Autodesk Inventor part; units mm, degrees
ref_plane "YZ Plane" through (0, 0, 0) normal (1, 0, 0) x (0, 1, 0)
ref_plane "XZ Plane" through (0, 0, 0) normal (0, 1, 0) x (-1, 0, 0)
ref_plane "XY Plane" through (0, 0, 0) normal (0, 0, 1) x (1, 0, 0)
sketch "Szkic2" plane through (0, 0, 0) normal (0, 1, 0) x (-1, 0, 0)
  line L0 (0, 0) -> (-15, 0) construction
  line L1 (-15, 0) -> (-15, 20)
  line L2 (-15, 20) -> (0, 20)
  line L3 (-15, 0) -> (-15, -20)
  line L4 (-15, -20) -> (0, -20)
  line L5 (0, -20) -> (0, 20) construction
  line L6 (15, 0) -> (15, 20)
  line L7 (15, 20) -> (0, 20)
  line L8 (15, -20) -> (0, -20)
  line L9 (15, 0) -> (15, -20)
  line L10 (15, 0) -> (13, 0) construction
  line L11 (0, 20) -> (0, 18) construction
  line L12 (0, 18) -> (13, 18)
  line L13 (13, 18) -> (13, 0)
  line L14 (0, 18) -> (-13, 18)
  line L15 (-13, 18) -> (-13, 0)
  line L16 (0, -18) -> (13, -18)
  line L17 (13, -18) -> (13, 0)
  line L18 (-13, -18) -> (-13, 0)
  line L19 (0, -18) -> (-13, -18)
  point P0 (-7.5, -20)
  point P1 (15, -10)
  dimension "d18" = 40
  dimension "d19" = 30
  dimension "d22" = 2
  dimension "d23" = 2
extrude "Wyciągnięcie proste4" add sketch "Szkic2" along normal blind 1200
sketch "Szkic3" plane through (15, 0, -20) normal (0, 0, -1) x (-1, 0, 0)
  line L0 (0, 1200) -> (0, 1180) construction
  line L1 (0, 0) -> (0, 1200)
  line L2 (0, 1180) -> (12, 1180) construction
  line L3 (12, 1180) -> (12, 0)
  line L4 (0, 0) -> (0, 1200)
  line L5 (0, 0) -> (0, 20)
  line L6 (0, 20) -> (12, 20)
  point P0 (15, 0)
  dimension "d26" = 20
  dimension "d27" = 12
  dimension "d76" = 1180
  dimension "d77" = 20
hole "Otwór1" at (3, 1180, -20) at (3, 20, -20) direction (0, 0, 1) diameter 8 depth 10 tip angle 118
sketch "Szkic4" plane through (15, 0, 20) normal (1, 0, 0) x (0, 0, -1)
  line L0 (40, 0) -> (0, 0)
  line L1 (0, 0) -> (10, 0)
  line L2 (40, 0) -> (30, 0)
  line L3 (0, 0) -> (0, 31)
  line L4 (0, 0) -> (0, 1200)
  line L5 (0, 31) -> (10, 31)
  line L6 (40, 0) -> (40, 1200)
  line L7 (40, 0) -> (40, 31)
  line L8 (30, 31) -> (40, 31)
  line L9 (40, 31) -> (40, 0)
  line L10 (0, 0) -> (0, 40)
  line L11 (20, 0) -> (20, 13)
  dimension "d35" = 10
  dimension "d36" = 10
  dimension "d37" = 31
  dimension "d38" = 20
  dimension "d39" = 31
  dimension "d40" = 10
  dimension "d41" = 40
  dimension "d42" = 13
hole "Otwór2" at (15, 31, 10) at (15, 31, -10) at (15, 13, 0) direction (-1, 0, 0) diameter 8 depth 8.25 tip angle 118
sketch "Szkic5" plane through (15, 0, 20) normal (1, 0, 0) x (0, 0, -1)
  line L0 (40, 0) -> (0, 0)
  line L1 (0, 0) -> (0, 45)
  line L2 (0, 0) -> (0, 1200)
  line L3 (0, 45) -> (20, 45)
  point P0 (20, 0)
  dimension "d50" = 45
hole "Otwór3" at (15, 45, 0) direction (-1, 0, 0) diameter 5 depth 8 tip angle 118
sketch "Szkic6" plane through (15, 0, 20) normal (1, 0, 0) x (0, 0, -1)
  line L0 (0, 0) -> (0, 1200)
  circle A0 centre (20, 45) radius 2.5
  line L1 (0, 45) -> (3, 45)
  line L2 (3, 45) -> (3, 245)
  line L3 (3, 245) -> (3, 445)
  line L4 (3, 445) -> (3, 645)
  line L5 (3, 645) -> (3, 845)
  line L6 (3, 845) -> (3, 1035)
  line L7 (40, 1200) -> (0, 1200)
  line L8 (20, 0) -> (20, 1200)
  line L9 (0, 1165) -> (4, 1165)
  point P0 (2, 1200)
  point P1 (37, 45)
  point P2 (37, 245)
  point P3 (37, 445)
  point P4 (37, 645)
  point P5 (37, 845)
  point P6 (37, 1035)
  point P7 (36, 1165)
  dimension "d58" = 20
  dimension "d59" = 3
  dimension "d60" = 200
  dimension "d61" = 200
  dimension "d62" = 200
  dimension "d63" = 200
  dimension "d64" = 190
  dimension "d73" = 35
  dimension "d75" = 4
hole "Otwór4" at (15, 45, 17) at (15, 245, 17) at (15, 445, 17) at (15, 645, 17) at (15, 845, 17) at (15, 1035, 17) at (15, 1165, 16) at (15, 1165, -16) at (15, 1035, -17) at (15, 845, -17) at (15, 645, -17) at (15, 445, -17) at (15, 245, -17) at (15, 45, -17) direction (-1, 0, 0) diameter 2.5 depth 8 tip angle 118
properties part number "profil_stalowy_40_30_120"
Here's how the part is built. I have some questions about the finished solid (model axes, mm). A direction names the side the tool comes from. Round coordinates to 2 decimals unless told otherwise and drop trailing zeros. Order: outer loops, then holes, each group sorted by start corner. A loop starts at its lowest first (then second) coordinate and runs counter-clockwise, first axis right, second up. Notation, with made-up numbers: M -5,-12.75 L 42,-12.75 A8 ccw 42,-3.75 Z; hole C -36.75,1 d9. An arc over 180 degrees is marked long. Return JSON: item names as keys, results as strings. Group by question number.
1. If we mould it in two halves opening along X, with no side actions, what happens to faces 3 (the face through (13.4, 0, 1.6)), 4 (the face through (-15, 592, 0)), 5 (the face through (0, 592, 18))? For each: pulls with the +X half, pulls with the -X half, needs draft (parallel to the pull), parting line crosses it, or undercut.
2. If we section it at B-B on y = 629.5: List the corners of the cut face in (x, z) for me.
3. If we section it at A-A on x = -5.5: List the corners of the cut face in (y, z) for me, then the cut area to 3 significant figures.
4. On a 3-axis mill with a long thin cutter (end or side, diameter ignored), from which of +Z, -Z, +X, -X, +Y, -Y can I reach the whole of each face in a straight line? I mean faces 1 (the face through (0, 592, -18)), 2 (the face through (0, 592, -20)). Say none if no direction works.
5. I'm going to push a flat-ended pin straight in: pin 1 Ø1.5 at (y, z) = (645, 17) entering from +X. Where does the tip first touch, or does it pass through?
6. Please list where these lines run through material, in increasing order: probe 1 along Z at (x, y) = (12.5, 946); probe 2 along Z at (x, y) = (10.75, 245); probe 3 along X at (y, z) = (597.5, 1).
Reply:
{
 "1": {"face 3": "needs draft", "face 4": "pulls with the -X half", "face 5": "undercut"},
 "2": {"outline": "M -15,-20 L 15,-20 L 15,20 L -15,20 Z; hole M -13,-18 L 13,-18 L 13,18 L -13,18 Z"},
 "3": {"outline": "M 0,-20 L 1200,-20 L 1200,-18 L 0,-18 Z; M 0,18 L 1200,18 L 1200,20 L 0,20 Z", "area": "4,800 mm^2"},
 "4": {"face 1": "+Y, -Y", "face 2": "-Z, +X, -X, +Y, -Y"},
 "5": {"pin 1": "x = -13"},
 "6": {"probe 1": "-20 to -18, 18 to 20", "probe 2": "-20 to -18.25, 18.25 to 20", "probe 3": "-15 to -13, 13 to 15"}
}
